```python
from build123d import *

# Parameters (mm, degrees)
MODEL_R             = 1.7499965
MODEL_R_2           = 1.6
BOSS_EXTRUDE1_DEPTH = 8
FILLET1_R           = 3
SKETCH1_R           = 0.875
SKETCH1_R_2         = 1.7499965
SKETCH1_R_3         = 1.6
BOSS_EXTRUDE2_DEPTH = 8
FILLET2_R           = 1
FILLET3_R           = 3
SKETCH2_R           = 2.9
CUT_EXTRUDE1_DEPTH  = 4
CHAMFER1_SIZE       = 1


with BuildPart() as part:
    # Model → Boss-Extrude1 (new body)
    with BuildSketch(Plane.XY):
        Polygon((20.40532142, 11.78), (-20.40532142, 11.78), (0, -23.563053444), align=None)
        with Locations((0, -16.5)):
            Circle(MODEL_R, mode=Mode.SUBTRACT)
        Circle(MODEL_R_2, mode=Mode.SUBTRACT)
        with Locations((-14.289419163, 8.25)):
            Circle(MODEL_R, mode=Mode.SUBTRACT)
        with Locations((14.289419163, 8.25)):
            Circle(MODEL_R, mode=Mode.SUBTRACT)
    extrude(amount=BOSS_EXTRUDE1_DEPTH)

    # Fillet1
    fillet1_edges = [part.edges().sort_by_distance(p)[0] for p in [
        (0, -23.563053444, 4),
        (-20.40532142, 11.78, 4),
        (20.40532142, 11.78, 4),
    ]]
    fillet(fillet1_edges, radius=FILLET1_R)

    # Sketch1 → Boss-Extrude2 (add)
    with BuildSketch(Plane(origin=(0, 0, 0), x_dir=(-1, 0, 0), z_dir=(0, 0, -1))):
        Polygon((-7, 16.58), (-7, 14), (-35.5, 14), (-35.5, -14), (-5.52123148, -14), (5.52123148, -14), (35.5, -14), (35.5, 14), (7, 14), (7, 16.58), align=None)
        with Locations((-1.5, 14.18)):
            Circle(SKETCH1_R, mode=Mode.SUBTRACT)
        with Locations((-4.5, 14.18)):
            Circle(SKETCH1_R, mode=Mode.SUBTRACT)
        with Locations((1.5, 14.18)):
            Circle(SKETCH1_R, mode=Mode.SUBTRACT)
        with Locations((4.5, 14.18)):
            Circle(SKETCH1_R, mode=Mode.SUBTRACT)
        with Locations(Location((-14.289419163, 8.25, 0), (0, 0, 180))):
            Circle(SKETCH1_R_2, mode=Mode.SUBTRACT)
        with Locations(Location((14.289419163, 8.25, 0), (0, 0, 180))):
            Circle(SKETCH1_R_2, mode=Mode.SUBTRACT)
        with Locations(Location((0, 0, 0), (0, 0, 180))):
            Circle(SKETCH1_R_3, mode=Mode.SUBTRACT)
        with BuildLine():
            Line((-27.5, 2), (-22.5, 2))
            ThreePointArc((-22.5, 2), (-20.5, 0), (-22.5, -2))
            Line((-22.5, -2), (-27.5, -2))
            ThreePointArc((-27.5, -2), (-29.5, 0), (-27.5, 2))
        make_face(mode=Mode.SUBTRACT)
        with BuildLine():
            Line((22.5, 2), (27.5, 2))
            ThreePointArc((27.5, 2), (29.5, 0), (27.5, -2))
            Line((27.5, -2), (22.5, -2))
            ThreePointArc((22.5, -2), (20.5, 0), (22.5, 2))
        make_face(mode=Mode.SUBTRACT)
    extrude(amount=-BOSS_EXTRUDE2_DEPTH)

    # Fillet2
    fillet2_edges = [part.edges().sort_by_distance(p)[0] for p in [
        (7, 16.58, 4),
        (-7, 16.58, 4),
        (-7, 14, 4),
        (7, 14, 4),
    ]]
    fillet(fillet2_edges, radius=FILLET2_R)

    # Fillet3
    fillet3_edges = [part.edges().sort_by_distance(p)[0] for p in [
        (-35.5, -14, 4),
        (-35.5, 14, 4),
        (35.5, -14, 4),
        (35.5, 14, 4),
    ]]
    fillet(fillet3_edges, radius=FILLET3_R)

    # Sketch2 → Cut-Extrude1 (cut)
    with BuildSketch(Plane.XY.offset(8)):
        with Locations((-14.289419163, 8.25)):
            Circle(SKETCH2_R)
        with Locations((14.289419163, 8.25)):
            Circle(SKETCH2_R)
        with Locations((0, -16.5)):
            Circle(SKETCH2_R)
    extrude(amount=-CUT_EXTRUDE1_DEPTH, mode=Mode.SUBTRACT)

    # Chamfer1
    chamfer1_edges = [part.edges().sort_by_distance(p)[0] for p in [
        (-1.6, 0, 0),
        (-16.039415663, 8.25, 0),
        (12.539422663, 8.25, 0),
        (-1.7499965, -16.5, 0),
    ]]
    chamfer(chamfer1_edges, length=CHAMFER1_SIZE)


solid = part.part
```
Here's how the part is built. I have some questions about the finished solid (model axes, mm). A direction names the side the tool comes from. Give positions to 0.01 mm unless a question says otherwise; leave off trailing zeros. Loops run counter-clockwise (first coordinate to the right, second up) from the corner with the lowest first, then second, coordinate; pieces in that order, holes last. Notation, with made-up numbers: M 23,77.25 L 56,77.25 A22 cw 56,114.25 Z; hole C 42,64.5 d5. An arc over 180 degrees is marked long. Put each result on its own line as item: value. Start each with the question number.
(1) For faces 1 (the cylindrical face through (16.97, 7.14, 6.03)), 2 (the cylindrical face through (-20.5, 0, 3.9)), 3 (the flat face through (0, -6, 0)), which set-ups out of +Z, -Z, +X, -X, +Y, -Y let a thin tool reach every point of the face, with its end or its side?
(2) I want a section at A-A on y = 0. Please give me the cut outline in (x, z), then the cut area to 3 significant figures.
(3) I want a section at C-C on y = 8.25. Please give me the cut outline in (x, z), then the cut area to 3 significant figures.
(4) Will these pins go through, and if not, where does the flat tip stop? pin 1 Ø2 at (x, y) = (-0.5, -0.5) entering from -Z; pin 2 Ø1.6 at (x, y) = (1.5, 14.18) entering from +Z; pin 3 Ø0.6 at (y, z) = (15, 4.5) entering from +X; pin 4 Ø4 at (x, z) = (-24, 6) entering from -Y.
(5) If we mould it in two halves opening along X, with no side actions, what happens to faces 4 (the cylindrical face through (-1.27, -0.97, 4.45)), 5 (the cylindrical face through (34.64, -13.1, 4.06)), 6 (the flat face through (-4.08, -16.5, 3.94))? For each: +X half, -X half, draft (parallel to the pull), parting line (faces both ways), or undercut.
(6) I need wall thicknesses on line 1 along X through (y, z) = (8, 4.5); line 2 along Y through (x, z) = (-26, 6.5); line 3 along Y through (x, z) = (17.5, 5.75). Which ranges of each line are inside material? Lowest first, please. Write a range as [from, to].
(7) I want a section at D-D on z = 7. State how many separate pieces and enclosed holes the cut face has, then the cut area to 3 significant figures.
(8) I want a section at B-B on x = 26.5. Please give me the cut outline in (y, z), then the cut area to 3 significant figures.
Answer block:
1. face 1: +Z
1. face 2: +Z, -Z
1. face 3: -Z, +X, -X, +Y, -Y
2. outline: M -35.5,0 L -29.5,0 L -29.5,8 L -35.5,8 Z; M -20.5,0 L -2.6,0 L -1.6,1 L -1.6,8 L -20.5,8 Z; M 1.6,1 L 2.6,0 L 20.5,0 L 20.5,8 L 1.6,8 Z; M 29.5,0 L 35.5,0 L 35.5,8 L 29.5,8 Z
2. area: 397 mm^2
3. outline: M -35.5,0 L -17.04,0 L -16.04,1 L -16.04,4 L -17.19,4 L -17.19,8 L -35.5,8 Z; M -12.54,1 L -11.54,0 L 11.54,0 L 12.54,1 L 12.54,4 L 11.39,4 L 11.39,8 L -11.39,8 L -11.39,4 L -12.54,4 Z; M 16.04,1 L 17.04,0 L 35.5,0 L 35.5,8 L 17.19,8 L 17.19,4 L 16.04,4 Z
3. area: 492 mm^2
4. pin 1: z = 0.89
4. pin 2: through
4. pin 3: x = 7.05
4. pin 4: y = -14
5. face 4: undercut
5. face 5: +X half
5. face 6: -X half
6. line 1: [-35.5, -17.18], [-11.4, 11.4], [17.18, 35.5]
6. line 2: [-14, -2], [2, 14]
6. line 3: [-14, 14]
7. separate pieces: 1
7. enclosed holes: 10
7. area: 1,900 mm^2
8. outline: M -14,0 L -2,0 L -2,8 L -14,8 Z; M 2,0 L 14,0 L 14,8 L 2,8 Z
8. area: 192 mm^2
